from build123d import *

# Parameters (mm, degrees)
F1_DEPTH = 4
F2_R     = 5
F3_DEPTH = 20
F4_R     = 0.5


with BuildPart() as f1:
    # F0 (on Top) → F1 (new body)
    with BuildSketch(Plane.XY):
        Polygon((8.554517, -1.349162), (5.445667, 6.733848), (-3.10885, 8.08301), (-8.554517, 1.349162), (-5.445667, -6.733848), (3.10885, -8.08301), align=None)
    extrude(amount=F1_DEPTH)

    # F2 (on face) → F3 (join)
    with BuildSketch(Plane.XY.offset(4)):
        Circle(F2_R)
    extrude(amount=F3_DEPTH)

    # F4
    f4_edges = [f1.edges().sort_by_distance(p)[0] for p in [
        (7.000092, 2.692343, 0),
        (1.168409, 7.408429, 0),
        (-5.831684, 4.716086, 0),
        (-7.000092, -2.692343, 0),
        (-1.168409, -7.408429, 0),
        (5.831684, -4.716086, 0),
        (8.554517, -1.349162, 2),
        (5.445667, 6.733848, 2),
        (-3.10885, 8.08301, 2),
        (3.10885, -8.08301, 2),
        (-8.554517, 1.349162, 2),
        (-5.445667, -6.733848, 2),
    ]]
    fillet(f4_edges, radius=F4_R)


solid = f1.part
Read the model definition and answer for the solid it produces. Units are mm, in the model's axes. A direction names the side the tool comes from. Coordinates: 2 decimals unless noted, no trailing zeros. Loops run counter-clockwise (first coordinate to the right, second up) from the corner with the lowest first, then second, coordinate; pieces in that order, holes last. Notation, with made-up numbers: (-22.5, 65) -> (8.5, 65) arc R26 cw to (8.5, 86) -> close; hole circle Ø2 at (64.5, -17). An arc over 180 degrees is marked (long way). Write item = value, one per line. Start each with the question number.
1) The part is cut by section A-A, the plane z = 12. Determine the outline of the cut face in (x, y), plus the area to 3 significant figures.
2) Given P1, Ø1, axis at y = 1.5, z = 11, coming from the -X side; P2, Ø3, axis at x = 5, y = -4.5, coming from the +Z side; P3, Ø2, axis at y = 3, z = 13, coming from the -X side, each flat-ended and moving along its own axis, determine where each tip first touches the part or whether it passes through.
3) Find the intervals of material crossed by L1, parallel to Z at x = -7, y = 0.5; L2, parallel to Y at x = -3, z = 11.25; L3, parallel to X at y = -1, z = 10.5, in increasing order. Write a range as from..to.
4) For faces 1 (the face through (6.85, 2.69, 0.15)), 2 (the face through (-3.9, -3.5, 4)), determine the directions among +Z, -Z, +X, -X, +Y, -Y from which every point of the face is accessible in a straight line to the end or side of a thin tool.
Result:
q1.outline = circle Ø10 at (0, 0)
q1.area = 78.5 mm²
q2.P1 = -4.9
q2.P2 = 4
q2.P3 = -4.58
q3.L1 = 0..4
q3.L2 = -4..4
q3.L3 = -4.9..4.9
q4.face_1 = -Z, +X, +Y
q4.face_2 = +Z
